```python
from build123d import *

# Parameters (mm, degrees)
SKETCH_1_W          = 560
SKETCH_1_H          = 60
SKETCH_1_R          = 10.25
SKETCH_1_R_2        = 2
EXTRUDE_1_DEPTH     = 4
SKETCH_2_R          = 2
CUT_EXTRUDE_1_DEPTH = 10
CUT_EXTRUDE_2_DEPTH = 10


with BuildPart() as part:
    # 草图1 → 凸台-拉伸1 (new body)
    with BuildSketch(Plane.XY):
        with Locations((250, 0)):
            Rectangle(SKETCH_1_W, SKETCH_1_H)
        Circle(SKETCH_1_R, mode=Mode.SUBTRACT)
        with Locations((0, -19)):
            Circle(SKETCH_1_R_2, mode=Mode.SUBTRACT)
        with Locations((-13.435028843, -13.435028843)):
            Circle(SKETCH_1_R_2, mode=Mode.SUBTRACT)
        with Locations((-19, 0)):
            Circle(SKETCH_1_R_2, mode=Mode.SUBTRACT)
        with Locations((-13.435028843, 13.435028843)):
            Circle(SKETCH_1_R_2, mode=Mode.SUBTRACT)
        with Locations((0, 19)):
            Circle(SKETCH_1_R_2, mode=Mode.SUBTRACT)
        with Locations((13.435028843, 13.435028843)):
            Circle(SKETCH_1_R_2, mode=Mode.SUBTRACT)
        with Locations((19, 0)):
            Circle(SKETCH_1_R_2, mode=Mode.SUBTRACT)
        with Locations((13.435028843, -13.435028843)):
            Circle(SKETCH_1_R_2, mode=Mode.SUBTRACT)
        with Locations((500, -19)):
            Circle(SKETCH_1_R_2, mode=Mode.SUBTRACT)
        with Locations((500, 0)):
            Circle(SKETCH_1_R, mode=Mode.SUBTRACT)
        with Locations((486.564971157, -13.435028843)):
            Circle(SKETCH_1_R_2, mode=Mode.SUBTRACT)
        with Locations((481, 0)):
            Circle(SKETCH_1_R_2, mode=Mode.SUBTRACT)
        with Locations((486.564971157, 13.435028843)):
            Circle(SKETCH_1_R_2, mode=Mode.SUBTRACT)
        with Locations((500, 19)):
            Circle(SKETCH_1_R_2, mode=Mode.SUBTRACT)
        with Locations((513.435028843, 13.435028843)):
            Circle(SKETCH_1_R_2, mode=Mode.SUBTRACT)
        with Locations((519, 0)):
            Circle(SKETCH_1_R_2, mode=Mode.SUBTRACT)
        with Locations((513.435028843, -13.435028843)):
            Circle(SKETCH_1_R_2, mode=Mode.SUBTRACT)
    extrude(amount=EXTRUDE_1_DEPTH)

    # 草图2 → 切除-拉伸1 (cut)
    with BuildSketch(Plane.XY.offset(4)):
        with Locations((-25, 25)):
            Circle(SKETCH_2_R)
        with Locations((53.5, 25)):
            Circle(SKETCH_2_R)
        with Locations((132, 25)):
            Circle(SKETCH_2_R)
        with Locations((210.5, 25)):
            Circle(SKETCH_2_R)
        with Locations((289, 25)):
            Circle(SKETCH_2_R)
        with Locations((367.5, 25)):
            Circle(SKETCH_2_R)
        with Locations((446, 25)):
            Circle(SKETCH_2_R)
        with Locations((524.5, 25)):
            Circle(SKETCH_2_R)
        with Locations((53.5, -25)):
            Circle(SKETCH_2_R)
        with Locations((132, -25)):
            Circle(SKETCH_2_R)
        with Locations((210.5, -25)):
            Circle(SKETCH_2_R)
        with Locations((289, -25)):
            Circle(SKETCH_2_R)
        with Locations((367.5, -25)):
            Circle(SKETCH_2_R)
        with Locations((446, -25)):
            Circle(SKETCH_2_R)
        with Locations((524.5, -25)):
            Circle(SKETCH_2_R)
        with Locations((-25, -25)):
            Circle(SKETCH_2_R)
    extrude(amount=-CUT_EXTRUDE_1_DEPTH, mode=Mode.SUBTRACT)

    # 草图3 → 切除-拉伸2 (cut)
    with BuildSketch(Plane.XY.offset(4)):
        Polygon((60, -18.5), (60, 18.5), (188.195742791, 18.5), (130.105742791, -18.5), align=None)
        Polygon((212.394257209, 18.5), (287.105742791, 18.5), (345.195742791, -18.5), (154.304257209, -18.5), align=None)
        Polygon((369.394257209, -18.5), (439.5, -18.5), (439.5, 18.5), (311.304257209, 18.5), align=None)
        Polygon((452.5, -12.369269395), (452.5, 12.369269395), (469.816977153, 0), align=None)
        Polygon((47, -12.262684635), (30.077495204, 0), (47, 12.262684635), align=None)
    extrude(amount=-CUT_EXTRUDE_2_DEPTH, mode=Mode.SUBTRACT)


solid = part.part
```
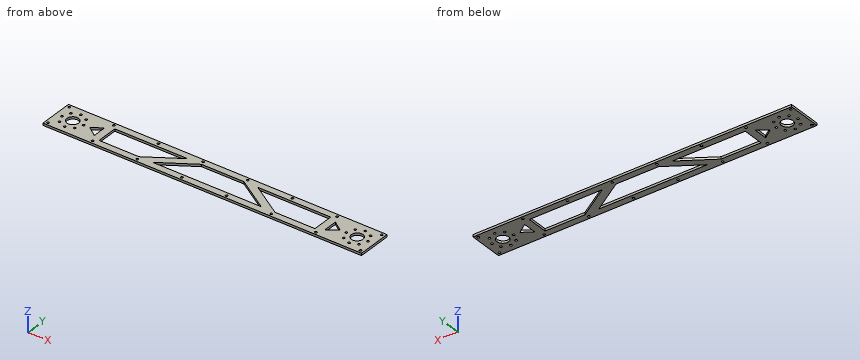
Work out the finished part from the listing and answer in its coordinate system (mm). Coordinates: 2 decimals unless noted, no trailing zeros. Loops run counter-clockwise (first coordinate to the right, second up) from the corner with the lowest first, then second, coordinate; pieces in that order, holes last. Notation, with made-up numbers: M 53.5,43.25 L 74.5,43.25 A19 ccw 74.5,53.25 Z; hole C 67,63.5 d2. An arc over 180 degrees is marked long. Use CSV: the item, a comma, the result in double quotes. Start each with the question number.
(1) Find section A-A, the plane x = 99. Give the vertices of the cut face in (y, z), then the cut area to 3 significant figures.
(2) Find section C-C, the plane x = 193. Give the vertices of the cut face in (y, z).
(3) Consider line 1 (Y direction, x = 446, z = 1.55); line 2 (Y direction, x = 405.5, z = 1.5); line 3 (Y direction, x = 289, z = 1.3). Determine where each line is inside the solid, lowest interval first.
(4) Find section B-B, the plane x = 332. Give the vertices of the cut face in (y, z).
(5) Find section D-D, the plane z = 0.7. State how many separate pieces and enclosed holes the cut face has, then the cut area to 3 significant figures.
Recorded:
1,outline,"M -30,0 L -18.5,0 L -18.5,4 L -30,4 Z; M 18.5,0 L 30,0 L 30,4 L 18.5,4 Z"
1,area,"92.0 mm^2"
2,outline,"M -30,0 L -18.5,0 L -18.5,4 L -30,4 Z; M 6.15,0 L 30,0 L 30,4 L 6.15,4 Z"
3,line 1,"y = -30 to -27, -23 to 23, 27 to 30"
3,line 2,"y = -30 to -18.5, 18.5 to 30"
3,line 3,"y = -30 to -27, -23 to -18.5, 17.29 to 23, 27 to 30"
4,outline,"M -30,0 L -18.5,0 L -18.5,4 L -30,4 Z; M -10.1,0 L 5.32,0 L 5.32,4 L -10.1,4 Z; M 18.5,0 L 30,0 L 30,4 L 18.5,4 Z"
5,separate pieces,"1"
5,enclosed holes,"39"
5,area,"19,900 mm^2"
